Design review of the part built by this model. Coordinates are the model's own, in mm. Face numbers are marked on the shaded views. A direction names the side the tool comes from. Give positions to 0.01 mm unless a question says otherwise; leave off trailing zeros. Order: outer loops, then holes, each group sorted by start corner. A loop starts at its lowest first (then second) coordinate and runs counter-clockwise, first axis right, second up. Notation, with made-up numbers: (-3, 30.25) -> (47, 30.25) arc R23 ccw to (47, 46.25) -> close; hole circle Ø8 at (83, 14.5). An arc over 180 degrees is marked (long way). One line per item, written item: value.
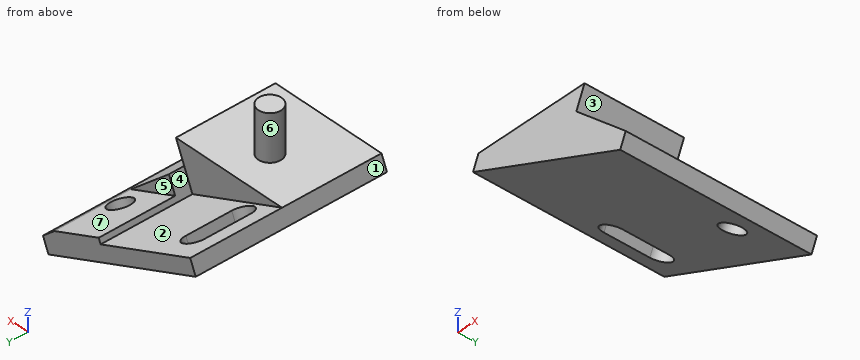
from build123d import *

# Parameters (mm, degrees)
PAD_DEPTH                      = 25
POCKET_DEPTH                   = 12
SKETCH002_R                    = 1.5
PAD001_DEPTH                   = 6
POCKET001_DEPTH                = 2.001
SKETCH004_W                    = 2.3
SKETCH004_H                    = 10
POCKET002_DEPTH                = 9.001
SKETCH005_R                    = 1.5
HOLE_DEPTH                     = 2.701
PART_MIRRORING_PLACEMENT_ANGLE = 23.19859


with BuildPart() as body:
    # Sketch → Pad (new body)
    with BuildSketch(Plane.XZ):
        Polygon((0, 0), (0, 2), (14, 8), (14, 5), (23, 2), (23, 0), align=None)
    extrude(amount=PAD_DEPTH)

    # Sketch001 (on Face8 of Pad) → Pocket (cut)
    with BuildSketch(Plane.XZ.offset(25)):
        Polygon((0, 2), (14, 2), (14, 8), align=None)
    extrude(amount=-POCKET_DEPTH, mode=Mode.SUBTRACT)

    # Sketch002 (on Face3 of Pocket) → Pad001 (join)
    with BuildSketch(Plane(origin=(-0.724138, 0, 1.689655), x_dir=(-0.919145, 0, -0.393919), z_dir=(-0.393919, 0, 0.919145))):
        with Locations((-8.019385, 8)):
            Circle(SKETCH002_R)
    extrude(amount=PAD001_DEPTH)

    # Sketch003 (on Face4 of Pad001) → Pocket001 (cut, through all)
    with BuildSketch(Plane(origin=(0, 0, 2), x_dir=(-1, 0, 0), z_dir=(0, 0, 1))):
        with BuildLine():
            ThreePointArc((-2.500319, 21.030919), (-4.030919, 22.499681), (-5.499681, 20.969081))
            Line((-5.499681, 14.969081), (-5.499681, 20.969081))
            ThreePointArc((-5.499681, 14.969081), (-3.969081, 13.500319), (-2.500319, 15.030919))
            Line((-2.500319, 15.030919), (-2.500319, 21.030919))
        make_face()
    extrude(amount=-POCKET001_DEPTH, mode=Mode.SUBTRACT)

    # Sketch004 (on Face15 of Pocket001) → Pocket002 (cut, through all)
    with BuildSketch(Plane(origin=(14, 0, 0), x_dir=(0, 0, -1), z_dir=(-1, 0, 0))):
        with Locations((-3.85, 20)):
            Rectangle(SKETCH004_W, SKETCH004_H)
    extrude(amount=-POCKET002_DEPTH, mode=Mode.SUBTRACT)

    # Sketch005 (on Face17 of Pocket002) → Hole (cut, through all)
    with BuildSketch(Plane(origin=(0, 0, 2.7), x_dir=(-1, 0, 0), z_dir=(0, 0, 1))):
        with Locations((-19, 18)):
            Circle(SKETCH005_R)
    extrude(amount=-HOLE_DEPTH, mode=Mode.SUBTRACT)


with BuildPart() as part_mirroring:
    # Part__Mirroring: instance of Body
    add(body.part.mirror(Plane(origin=(0, 0, 0), x_dir=(1, 0, 0), z_dir=(0, 1, 0))))


with BuildPart() as part_mirroring_1:
    # Part__Mirroring placement: moved
    add(part_mirroring.part.moved(Location((-8.019385, -8, -3.338294))).rotate(Axis((-8.019385, -8, -3.338294), (0, 1, 0)), PART_MIRRORING_PLACEMENT_ANGLE))


solid = part_mirroring_1.part
Item 1: Add section A-A on y = 0. Give the boundary of the cut face in (x, z).
Returned:
outline: (-8.02, -3.34) -> (13.12, -12.4) -> (13.91, -10.56) -> (6.82, -4.26) -> (8, -1.5) -> (1.5, -1.5) -> (1.5, 4.5) -> (-1.5, 4.5) -> (-1.5, -1.5) -> (-7.23, -1.5) -> close
Item 2: Clearance check with flat-ended pins moving along their axes: P1, Ø12, axis at x = -5, y = 13, coming from the +Z side; P2, Ø4, axis at x = -1.5, z = 2, coming from the +Y side; P3, Ø3, axis at x = 9, y = 11.5, coming from the -Z side; P4, Ø4, axis at x = -5, z = -6.5, coming from the -Y side. State where each tip first meets the part, or that it passes through.
Returned:
P1: z = -1.5
P2: y = 1.5
P3: z = -11.28
P4: y = -8
Item 3: To check wall thickness, follow line 1 along Y through (x, z) = (5.75, -4); line 2 along X through (y, z) = (-3.5, -7.75); line 3 along Y through (x, z) = (9.5, -10.25). State the ranges of each line that lie inside material, in increasing order. Write a range as from..to.
Returned:
line 1: -8..5
line 2: 2.27..10.75
line 3: -8..8.51, 11.49..17
Item 4: Add section B-B on x = 3. Give the boundary of the cut face in (y, z).
Returned:
outline: (-8, -8.06) -> (17, -8.06) -> (17, -5.88) -> (5, -5.88) -> (5, -1.5) -> (-8, -1.5) -> close
Item 5: Draft analysis for pull direction X (two halves, no side actions). For the marked faces 4, 5, 6 and 7, state which applies: pulls with the +X half, pulls with the -X half, needs draft (parallel to the pull), parting line crosses it, or undercut.
Returned:
face 4: undercut
face 5: needs draft
face 6: parting line crosses it
face 7: pulls with the +X half
Item 6: Machinability: for the marked faces 1, 2 and 3, which of the approach directions +Z, -Z, +X, -X, +Y, -Y give a long, thin tool a straight path to every point of the face, cutting with its end or side? Answer none if there is none.
Returned:
face 1: +Z, -X, +Y, -Y
face 2: +Z, +Y
face 3: +X, +Y, -Y
